Autodesk Inventor part; units mm, degrees
ref_plane "YZ Plane" through (0, 0, 0) normal (1, 0, 0) x (0, 1, 0)
ref_plane "XZ Plane" through (0, 0, 0) normal (0, 1, 0) x (-1, 0, 0)
ref_plane "XY Plane" through (0, 0, 0) normal (0, 0, 1) x (1, 0, 0)
sketch "Sketch1" plane through (0, 0, 0) normal (0, 0, 1) x (1, 0, 0)
  line L0 (-15.875, 14.2748) -> (-15.875, -14.2748)
  arc A0 (-14.2748, 15.875) -> (-15.875, 14.2748) centre (-14.2748, 14.2748) ccw
  line L1 (14.2748, 15.875) -> (-14.2748, 15.875)
  arc A1 (15.875, 14.2748) -> (14.2748, 15.875) centre (14.2748, 14.2748) ccw
  line L2 (15.875, -14.2748) -> (15.875, 14.2748)
  arc A2 (14.2748, -15.875) -> (15.875, -14.2748) centre (14.2748, -14.2748) ccw
  line L3 (-14.2748, -15.875) -> (14.2748, -15.875)
  arc A3 (-15.875, -14.2748) -> (-14.2748, -15.875) centre (-14.2748, -14.2748) ccw
  arc A4 (19.05, 15.875) -> (15.875, 19.05) centre (15.875, 15.875) ccw
  line L4 (15.875, 19.05) -> (-15.875, 19.05)
  arc A5 (-15.875, 19.05) -> (-19.05, 15.875) centre (-15.875, 15.875) ccw
  line L5 (-19.05, 15.875) -> (-19.05, -15.875)
  arc A6 (-19.05, -15.875) -> (-15.875, -19.05) centre (-15.875, -15.875) ccw
  line L6 (-15.875, -19.05) -> (15.875, -19.05)
  arc A7 (15.875, -19.05) -> (19.05, -15.875) centre (15.875, -15.875) ccw
  line L7 (19.05, -15.875) -> (19.05, 15.875)
  point P0 (0, 0)
extrude "Extrusion1" add sketch "Sketch1" against normal blind 304.8
hole "Hole1" at (19.05, -1.5802, -19.05) direction (-1, 0, 0) diameter 8.3312 end through all
hole "Hole2" at (0, 19.05, -19.05) direction (0, -1, 0) diameter 8.3312 end through all
pattern_linear "Rectangular Pattern1" count 180 spacing 38.1 along (0, 0, -1) of "Hole2", "Hole1"
properties part number "9701"
Part model, mm, in its own coordinate system. Give positions to 0.01 mm unless a question says otherwise; leave off trailing zeros. Loops run counter-clockwise (first coordinate to the right, second up) from the corner with the lowest first, then second, coordinate; pieces in that order, holes last. Notation, with made-up numbers: M 64.25,20 L 123.25,20 A17 cw 123.25,51 Z; hole C 65.5,-6 d8. An arc over 180 degrees is marked long. Put each result on its own line as item: value. Start each with the question number.
1) Probe probe 1 along X at (y, z) = (-8.5, -27.5) (3 decimals); probe 2 along X at (y, z) = (17.95, -19.05). List the from-to ranges inside material, lowest first.
2) Pull direction Z, two halves, no side cores. Call faces 1 (the cylindrical face through (-17.485, 0.015, -251.498)), 2 (the flat face through (-17, 0, 0)), 3 (the flat face through (0, -15.875, -150)): +Z half, -Z half, draft (parallel to the pull), parting line (faces both ways), or undercut.
3) Saw through at A-A (z = -95.25). State how many separate pieces and enclosed holes the cut face has, then the cut area to 3 significant figures.
4) Saw through at C-C (z = -220). List the corners of the cut face in (x, y) (3 decimals).
5) Saw through at B-B (x = -10.5). List the corners of the cut face in (y, z) (3 decimals), then the cut area to 3 significant figures.
Numbers:
1. probe 1: -19.05 to -15.875, 15.875 to 19.05
1. probe 2: -18.28 to -4.17, 4.17 to 18.28
2. face 1: undercut
2. face 2: +Z half
2. face 3: draft
3. separate pieces: 4
3. enclosed holes: 0
3. area: 331 mm^2
4. outline: M -19.05,-15.875 A3.175 ccw -15.875,-19.05 L 15.875,-19.05 A3.175 ccw 19.05,-15.875 L 19.05,15.875 A3.175 ccw 15.875,19.05 L -15.875,19.05 A3.175 ccw -19.05,15.875 Z; hole M -15.875,-14.275 A1.6 ccw -14.275,-15.875 L 14.275,-15.875 A1.6 ccw 15.875,-14.275 L 15.875,14.275 A1.6 ccw 14.275,15.875 L -14.275,15.875 A1.6 ccw -15.875,14.275 Z
5. outline: M -19.05,-304.8 L -15.875,-304.8 L -15.875,0 L -19.05,0 Z; M 15.875,-304.8 L 19.05,-304.8 L 19.05,0 L 15.875,0 Z
5. area: 1,940 mm^2
